```python
from build123d import *

# Parameters (mm, degrees)
SKETCH1_W           = 25
SKETCH1_H           = 16.5
BOSS_EXTRUDE1_DEPTH = 2.88
SKETCH2_R           = 1
CUT_EXTRUDE1_DEPTH  = 18.565431962
FILLET1_R           = 2


with BuildPart() as part:
    # Sketch1 → Boss-Extrude1 (new body)
    with BuildSketch(Plane(origin=(0, 0, 0), x_dir=(1, 0, 0), z_dir=(0, 1, 0))):
        with Locations((0, -3.75)):
            Rectangle(SKETCH1_W, SKETCH1_H)
    extrude(amount=BOSS_EXTRUDE1_DEPTH)

    # Sketch2 → Cut-Extrude1 (cut, through all)
    with BuildSketch(Plane(origin=(0, 2.88, 0), x_dir=(1, 0, 0), z_dir=(0, 1, 0))):
        with Locations(Location((-10.5, 2.5, 0), (0, 0, 270))):
            Circle(SKETCH2_R)
        with Locations(Location((-10.5, -10, 0), (0, 0, 270))):
            Circle(SKETCH2_R)
        with Locations(Location((10.5, -10, 0), (0, 0, 270))):
            Circle(SKETCH2_R)
        with Locations(Location((10.5, 2.5, 0), (0, 0, 270))):
            Circle(SKETCH2_R)
    extrude(amount=-CUT_EXTRUDE1_DEPTH, mode=Mode.SUBTRACT)

    # Fillet1
    fillet1_edges = [part.edges().sort_by_distance(p)[0] for p in [
        (12.5, 1.44, 12),
        (-12.5, 1.44, 12),
    ]]
    fillet(fillet1_edges, radius=FILLET1_R)


solid = part.part
```
Source: CAD feature listing. Evaluate the final solid. Frame: model axes, mm. Give positions to 0.01 mm unless a question says otherwise; leave off trailing zeros. Write each loop counter-clockwise with the first axis right and the second up, starting at its lowest first coordinate (ties: lowest second). Pieces come first, ordered by that corner, then holes.
1. Material intervals for line 1 along X through (y, z) = (1.55, 10); line 2 along Z through (x, y) = (-11.25, 1), sorted ascending.
2. Pull-direction query (X, two-part tool) for faces 1 (the face through (11.9, 1.46, 11.43)), 2 (the face through (0, 2.88, 4)), 3 (the face through (-9.51, 1.46, 9.87)); classes: +X half, -X half, draft (parallel to the pull), parting line (faces both ways), or undercut.
3. Section query B-B (y = 1.25). Return the cut outline in (x, z).
4. Section query A-A (z = -2.5). Return the cut outline in (x, y).
5. Section query C-C (x = 9.75). Return the cut outline in (y, z), then the cut area to 3 significant figures.
6. First-contact query: pin 1 (2 mm diameter, centred on x = 5, z = 4, fed in from -Y). Flat tip, straight axial feed; report the tip coordinate or a pass-through.
Output values:
1. line 1: x = -12.5 to -11.5, -9.5 to 9.5, 11.5 to 12.5
1. line 2: z = -4.5 to -3.16, -1.84 to 9.34, 10.66 to 11.85
2. face 1: +X half
2. face 2: draft
2. face 3: undercut
3. outline: (-12.5, -4.5) - (12.5, -4.5) - (12.5, 10) arc R2 ccw to (10.5, 12) - (-10.5, 12) arc R2 ccw to (-12.5, 10) - close; hole circle Ø2 at (-10.5, -2.5); hole circle Ø2 at (-10.5, 10); hole circle Ø2 at (10.5, -2.5); hole circle Ø2 at (10.5, 10)
4. outline: (-12.5, 0) - (-11.5, 0) - (-11.5, 2.88) - (-12.5, 2.88) - close; (-9.5, 0) - (9.5, 0) - (9.5, 2.88) - (-9.5, 2.88) - close; (11.5, 0) - (12.5, 0) - (12.5, 2.88) - (11.5, 2.88) - close
5. outline: (0, -4.5) - (2.88, -4.5) - (2.88, -3.16) - (0, -3.16) - close; (0, -1.84) - (2.88, -1.84) - (2.88, 9.34) - (0, 9.34) - close; (0, 10.66) - (2.88, 10.66) - (2.88, 12) - (0, 12) - close
5. area: 39.9 mm2
6. pin 1: stops at y = 0
